from build123d import *

# Parameters (mm, degrees)
CROQUIS1_W              = 20
CROQUIS1_H              = 42
SALIENTE_EXTRUIR1_DEPTH = 3.175
CROQUIS2_R              = 3.175
SALIENTE_EXTRUIR2_DEPTH = 12
CROQUIS3_W              = 12
CROQUIS3_H              = 35
SALIENTE_EXTRUIR3_DEPTH = 13
CROQUIS4_R              = 3.175
SALIENTE_EXTRUIR4_DEPTH = 11
SALIENTE_EXTRUIR5_START = 11
CROQUIS5_R              = 3.175
SALIENTE_EXTRUIR5_DEPTH = 11
SALIENTE_EXTRUIR6_START = -6
CROQUIS6_R              = 10
CROQUIS6_R_2            = 3.175
SALIENTE_EXTRUIR6_DEPTH = 6
CROQUIS7_R              = 10
CROQUIS7_R_2            = 3.175
SALIENTE_EXTRUIR7_DEPTH = 6


with BuildPart() as part:
    # Croquis1 → Saliente-Extruir1 (new body)
    with BuildSketch(Plane(origin=(0, 0, 0), x_dir=(1, 0, 0), z_dir=(0, 1, 0))):
        with Locations((10, -21)):
            Rectangle(CROQUIS1_W, CROQUIS1_H)
    extrude(amount=SALIENTE_EXTRUIR1_DEPTH)

    # Croquis2 → Saliente-Extruir2 (add)
    with BuildSketch(Plane(origin=(0, 3.175, 0), x_dir=(1, 0, 0), z_dir=(0, 1, 0))):
        with Locations(Location((10, -21, 0), (0, 0, 270))):
            Circle(CROQUIS2_R)
    extrude(amount=SALIENTE_EXTRUIR2_DEPTH)

    # Croquis3 → Saliente-Extruir3 (add)
    with BuildSketch(Plane(origin=(0, 15.175, 0), x_dir=(1, 0, 0), z_dir=(0, 1, 0))):
        with Locations((10, -21)):
            Rectangle(CROQUIS3_W, CROQUIS3_H)
    extrude(amount=SALIENTE_EXTRUIR3_DEPTH)

    # Croquis4 → Saliente-Extruir4 (add)
    with BuildSketch(Plane.ZY.offset(-4)):
        with Locations(Location((9.5, 21.675, 0), (0, 0, 180))):
            Circle(CROQUIS4_R)
        with Locations(Location((32.5, 21.675, 0), (0, 0, 180))):
            Circle(CROQUIS4_R)
    extrude(amount=SALIENTE_EXTRUIR4_DEPTH)

    # Croquis5 → Saliente-Extruir5 (add)
    with BuildSketch(Plane(origin=(16, 0, 0), x_dir=(0, 0, -1), z_dir=(1, 0, 0)).offset(SALIENTE_EXTRUIR5_START)):
        with Locations((-32.5, 21.675)):
            Circle(CROQUIS5_R)
        with Locations((-9.5, 21.675)):
            Circle(CROQUIS5_R)
    extrude(amount=-SALIENTE_EXTRUIR5_DEPTH)

    # Croquis6 → Saliente-Extruir6 (add)
    # profile 1 of 2: a face of its own
    with BuildSketch(Plane.ZY.offset(7).offset(SALIENTE_EXTRUIR6_START)):
        with Locations((9.5, 21.675)):
            Circle(CROQUIS6_R)
        with Locations(Location((9.5, 21.675, 0), (0, 0, 180))):
            Circle(CROQUIS6_R_2, mode=Mode.SUBTRACT)
    # profile 2 of 2: a face of its own
    with BuildSketch(Plane.ZY.offset(7).offset(SALIENTE_EXTRUIR6_START)):
        with Locations((32.5, 21.675)):
            Circle(CROQUIS6_R)
        with Locations(Location((32.5, 21.675, 0), (0, 0, 180))):
            Circle(CROQUIS6_R_2, mode=Mode.SUBTRACT)
    extrude(amount=SALIENTE_EXTRUIR6_DEPTH)

    # Croquis7 → Saliente-Extruir7 (add)
    # profile 1 of 2: a face of its own
    with BuildSketch(Plane(origin=(27, 0, 0), x_dir=(0, 0, -1), z_dir=(1, 0, 0))):
        with Locations(Location((-32.5, 21.675, 0), (0, 0, 180))):
            Circle(CROQUIS7_R)
        with Locations(Location((-32.5, 21.675, 0), (0, 0, 180))):
            Circle(CROQUIS7_R_2, mode=Mode.SUBTRACT)
    # profile 2 of 2: a face of its own
    with BuildSketch(Plane(origin=(27, 0, 0), x_dir=(0, 0, -1), z_dir=(1, 0, 0))):
        with Locations(Location((-9.5, 21.675, 0), (0, 0, 180))):
            Circle(CROQUIS7_R)
        with Locations(Location((-9.5, 21.675, 0), (0, 0, 180))):
            Circle(CROQUIS7_R_2, mode=Mode.SUBTRACT)
    extrude(amount=-SALIENTE_EXTRUIR7_DEPTH)


solid = part.part
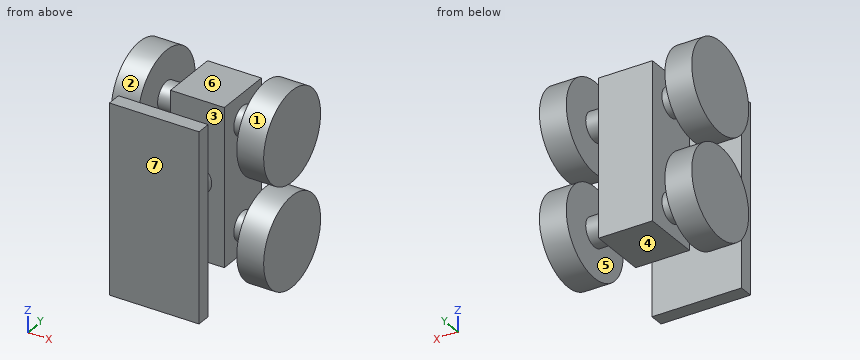
For this review, take the finished solid that the model builds, in its own axes (mm). Face numbers are marked on the shaded views. A direction names the side the tool comes from. Round coordinates to 2 decimals unless told otherwise and drop trailing zeros. Loops run counter-clockwise (first coordinate to the right, second up) from the corner with the lowest first, then second, coordinate; pieces in that order, holes last. Notation, with made-up numbers: (85.5, 82.25) - (120.5, 82.25) arc R23 cw to (120.5, 94.25) - close; hole circle Ø8 at (40, 50). An arc over 180 degrees is marked (long way). Use one line per item in the form item = value.
1) Tool access review of the marked faces 1, 2 and 3: name each direction out of +Z, -Z, +X, -X, +Y, -Y from which nothing blocks a thin tool from reaching the whole face with its end or side.
Solutions:
face_1 = +X
face_2 = -X
face_3 = none
2) Clearance check with flat-ended pins moving along their axes: P1, Ø13, axis at x = 10, y = 20, coming from the -Z side; P2, Ø12, axis at x = 15, y = 6, coming from the -Z side; P3, Ø2.5, axis at y = 1, z = 13.5, coming from the +X side. State where each tip first meets the part, or that it passes through.
Solutions:
P1 = 3.5
P2 = 0
P3 = 20
3) Wall thickness on probe 1 along X at (y, z) = (26.5, 10); probe 2 along X at (y, z) = (30, 13); probe 3 along Y at (x, z) = (7, 37) (3 decimals): over which ranges is each line inside the solid? List them lowest first.
Solutions:
probe_1 = -7 to -1, 4 to 16, 21 to 27
probe_2 = -7 to -1, 21 to 27
probe_3 = 0 to 3.175, 15.175 to 28.175
4) We need section A-A on z = 9.5. Write out the cut boundary in (x, y) (3 decimals), then the cut area to 3 significant figures.
Solutions:
outline = (-7, 11.675) - (-1, 11.675) - (-1, 18.5) - (4, 18.5) - (4, 15.175) - (16, 15.175) - (16, 18.5) - (21, 18.5) - (21, 11.675) - (27, 11.675) - (27, 31.675) - (21, 31.675) - (21, 24.85) - (16, 24.85) - (16, 28.175) - (4, 28.175) - (4, 24.85) - (-1, 24.85) - (-1, 31.675) - (-7, 31.675) - close; (0, 0) - (20, 0) - (20, 3.175) - (0, 3.175) - close
area = 523 mm2
5) We need section D-D on x = 18. Write out the cut boundary in (y, z) (3 decimals).
Solutions:
outline = (0, 0) - (3.175, 0) - (3.175, 42) - (0, 42) - close; circle Ø6.35 at (21.675, 9.5); circle Ø6.35 at (21.675, 32.5)
6) We need section B-B on x = 10. Write out the cut boundary in (y, z) (3 decimals), then the cut area to 3 significant figures.
Solutions:
outline = (0, 0) - (3.175, 0) - (3.175, 17.825) - (15.175, 17.825) - (15.175, 3.5) - (28.175, 3.5) - (28.175, 38.5) - (15.175, 38.5) - (15.175, 24.175) - (3.175, 24.175) - (3.175, 42) - (0, 42) - close
area = 665 mm2
7) We need section C-C on z = 36.5. Write out the cut boundary in (x, y) (3 decimals), then the cut area to 3 significant figures.
Solutions:
outline = (-7, 12.51) - (-1, 12.51) - (-1, 30.84) - (-7, 30.84) - close; (0, 0) - (20, 0) - (20, 3.175) - (0, 3.175) - close; (4, 15.175) - (16, 15.175) - (16, 28.175) - (4, 28.175) - close; (21, 12.51) - (27, 12.51) - (27, 30.84) - (21, 30.84) - close
area = 439 mm2
8) Mouldability with a two-part tool opening along Z and no side actions: class the marked faces 4, 5, 6 and 7 as pulls with the +Z half, pulls with the -Z half, needs draft (parallel to the pull), parting line crosses it, or undercut.
Solutions:
face_4 = pulls with the -Z half
face_5 = undercut
face_6 = pulls with the +Z half
face_7 = needs draft
